Geometry: final body of the model. Coordinates: model frame, mm. A direction names the side the tool comes from. Coordinates: 2 decimals unless noted, no trailing zeros. Write each loop counter-clockwise with the first axis right and the second up, starting at its lowest first coordinate (ties: lowest second). Pieces come first, ordered by that corner, then holes. Notation, with made-up numbers: (-36.75, 33.5) -> (-28.75, 33.5) arc R33 cw to (-28.75, 71.5) -> close; hole circle Ø9 at (-35, 75.5). An arc over 180 degrees is marked (long way). One line per item, written item: value.
```python
from build123d import *

# Parameters (mm, degrees)
SKETCH1_R           = 1.5
SKETCH1_R_2         = 1.6
SKETCH1_R_3         = 2.55
SKETCH1_R_4         = 2.1
BOSS_EXTRUDE1_DEPTH = 6.25


with BuildPart() as part:
    # Sketch1 → Boss-Extrude1 (new body)
    with BuildSketch(Plane.XY):
        Polygon((180, 196.75), (-180, 196.75), (-185, 191.75), (-185, -168.25), (-180, -173.25), (-160, -173.25), (-156, -169.25), (-148, -169.25), (-144, -173.25), (-63, -173.25), (-58, -168.25), (-39, -168.25), (-34, -173.25), (144, -173.25), (148, -169.25), (156, -169.25), (160, -173.25), (180, -173.25), (185, -168.25), (185, 191.75), align=None)
        with Locations(Location((165, -153.45, 0), (0, 0, 180))):  # turned: the seam where the file's is
            Circle(SKETCH1_R, mode=Mode.SUBTRACT)
        with Locations(Location((-155, 186.55, 0), (0, 0, 180))):  # turned: the seam where the file's is
            Circle(SKETCH1_R, mode=Mode.SUBTRACT)
        with Locations(Location((-175, -133.45, 0), (0, 0, 180))):  # turned: the seam where the file's is
            Circle(SKETCH1_R, mode=Mode.SUBTRACT)
        with Locations(Location((-65, -143.25, 0), (0, 0, 180))):  # turned: the seam where the file's is
            Circle(SKETCH1_R_2, mode=Mode.SUBTRACT)
        with Locations(Location((-175, 186.55, 0), (0, 0, 180))):  # turned: the seam where the file's is
            Circle(SKETCH1_R, mode=Mode.SUBTRACT)
        with Locations(Location((-180.1, -11.45, 0), (0, 0, 180))):  # turned: the seam where the file's is
            Circle(SKETCH1_R, mode=Mode.SUBTRACT)
        with Locations(Location((-181.5, 96.05, 0), (0, 0, 180))):  # turned: the seam where the file's is
            Circle(SKETCH1_R, mode=Mode.SUBTRACT)
        with Locations(Location((-181.3, 7.85, 0), (0, 0, 180))):  # turned: the seam where the file's is
            Circle(SKETCH1_R, mode=Mode.SUBTRACT)
        with Locations(Location((-138, 1.45, 0), (0, 0, 180))):  # turned: the seam where the file's is
            Circle(SKETCH1_R, mode=Mode.SUBTRACT)
        with Locations(Location((-138.5, 96.05, 0), (0, 0, 180))):  # turned: the seam where the file's is
            Circle(SKETCH1_R, mode=Mode.SUBTRACT)
        with Locations(Location((-165, -153.45, 0), (0, 0, 180))):  # turned: the seam where the file's is
            Circle(SKETCH1_R, mode=Mode.SUBTRACT)
        with Locations(Location((-181.3, -73.45, 0), (0, 0, 180))):  # turned: the seam where the file's is
            Circle(SKETCH1_R, mode=Mode.SUBTRACT)
        with Locations(Location((175, 186.55, 0), (0, 0, 180))):  # turned: the seam where the file's is
            Circle(SKETCH1_R, mode=Mode.SUBTRACT)
        with Locations(Location((-170, 74.55, 0), (0, 0, 180))):  # turned: the seam where the file's is
            Circle(SKETCH1_R, mode=Mode.SUBTRACT)
        with Locations(Location((-138, -73.45, 0), (0, 0, 180))):  # turned: the seam where the file's is
            Circle(SKETCH1_R, mode=Mode.SUBTRACT)
        with Locations(Location((155, -133.45, 0), (0, 0, 180))):  # turned: the seam where the file's is
            Circle(SKETCH1_R, mode=Mode.SUBTRACT)
        with Locations(Location((175, -133.45, 0), (0, 0, 180))):  # turned: the seam where the file's is
            Circle(SKETCH1_R, mode=Mode.SUBTRACT)
        with Locations(Location((-180.1, -105.45, 0), (0, 0, 180))):  # turned: the seam where the file's is
            Circle(SKETCH1_R, mode=Mode.SUBTRACT)
        with Locations(Location((155, 186.55, 0), (0, 0, 180))):  # turned: the seam where the file's is
            Circle(SKETCH1_R, mode=Mode.SUBTRACT)
        with Locations(Location((-170, 117.55, 0), (0, 0, 180))):  # turned: the seam where the file's is
            Circle(SKETCH1_R, mode=Mode.SUBTRACT)
        with Locations(Location((-159, -166.25, 0), (0, 0, 180))):  # turned: the seam where the file's is
            Circle(SKETCH1_R_2, mode=Mode.SUBTRACT)
        with Locations(Location((133.6, -168.35, 0), (0, 0, 180))):  # turned: the seam where the file's is
            Circle(SKETCH1_R_3, mode=Mode.SUBTRACT)
        with Locations(Location((-145, -166.25, 0), (0, 0, 180))):  # turned: the seam where the file's is
            Circle(SKETCH1_R_2, mode=Mode.SUBTRACT)
        with Locations(Location((96.6, -145.15, 0), (0, 0, 180))):  # turned: the seam where the file's is
            Circle(SKETCH1_R_3, mode=Mode.SUBTRACT)
        with Locations(Location((73.4, -168.35, 0), (0, 0, 180))):  # turned: the seam where the file's is
            Circle(SKETCH1_R_3, mode=Mode.SUBTRACT)
        with Locations(Location((-73.4, -168.35, 0), (0, 0, 180))):  # turned: the seam where the file's is
            Circle(SKETCH1_R_3, mode=Mode.SUBTRACT)
        with Locations(Location((96.6, -168.35, 0), (0, 0, 180))):  # turned: the seam where the file's is
            Circle(SKETCH1_R_3, mode=Mode.SUBTRACT)
        with Locations(Location((-73.4, -145.15, 0), (0, 0, 180))):  # turned: the seam where the file's is
            Circle(SKETCH1_R_3, mode=Mode.SUBTRACT)
        with Locations(Location((-110.4, -168.35, 0), (0, 0, 180))):  # turned: the seam where the file's is
            Circle(SKETCH1_R_3, mode=Mode.SUBTRACT)
        with Locations(Location((-133.6, -168.35, 0), (0, 0, 180))):  # turned: the seam where the file's is
            Circle(SKETCH1_R_3, mode=Mode.SUBTRACT)
        with Locations(Location((-110.4, -145.15, 0), (0, 0, 180))):  # turned: the seam where the file's is
            Circle(SKETCH1_R_3, mode=Mode.SUBTRACT)
        with Locations(Location((73.4, -145.15, 0), (0, 0, 180))):  # turned: the seam where the file's is
            Circle(SKETCH1_R_3, mode=Mode.SUBTRACT)
        with Locations(Location((146, -166.25, 0), (0, 0, 180))):  # turned: the seam where the file's is
            Circle(SKETCH1_R_2, mode=Mode.SUBTRACT)
        with Locations(Location((-133.6, -145.15, 0), (0, 0, 180))):  # turned: the seam where the file's is
            Circle(SKETCH1_R_3, mode=Mode.SUBTRACT)
        with Locations(Location((110.4, -145.15, 0), (0, 0, 180))):  # turned: the seam where the file's is
            Circle(SKETCH1_R_3, mode=Mode.SUBTRACT)
        with Locations(Location((-96.6, -145.15, 0), (0, 0, 180))):  # turned: the seam where the file's is
            Circle(SKETCH1_R_3, mode=Mode.SUBTRACT)
        with Locations(Location((110.4, -168.35, 0), (0, 0, 180))):  # turned: the seam where the file's is
            Circle(SKETCH1_R_3, mode=Mode.SUBTRACT)
        with Locations(Location((133.6, -145.15, 0), (0, 0, 180))):  # turned: the seam where the file's is
            Circle(SKETCH1_R_3, mode=Mode.SUBTRACT)
        with Locations(Location((-96.6, -168.35, 0), (0, 0, 180))):  # turned: the seam where the file's is
            Circle(SKETCH1_R_3, mode=Mode.SUBTRACT)
        with Locations(Location((158, -166.25, 0), (0, 0, 180))):  # turned: the seam where the file's is
            Circle(SKETCH1_R_2, mode=Mode.SUBTRACT)
        with Locations(Location((-65, -160.25, 0), (0, 0, 180))):  # turned: the seam where the file's is
            Circle(SKETCH1_R_2, mode=Mode.SUBTRACT)
        with Locations(Location((-65, -169.25, 0), (0, 0, 180))):  # turned: the seam where the file's is
            Circle(SKETCH1_R_2, mode=Mode.SUBTRACT)
        with Locations(Location((45, -160.25, 0), (0, 0, 180))):  # turned: the seam where the file's is
            Circle(SKETCH1_R_2, mode=Mode.SUBTRACT)
        with Locations(Location((148.4, 31.75, 0), (0, 0, 180))):  # turned: the seam where the file's is
            Circle(SKETCH1_R_4, mode=Mode.SUBTRACT)
        with Locations(Location((45, -169.25, 0), (0, 0, 180))):  # turned: the seam where the file's is
            Circle(SKETCH1_R_2, mode=Mode.SUBTRACT)
        with Locations(Location((148.4, -85.25, 0), (0, 0, 180))):  # turned: the seam where the file's is
            Circle(SKETCH1_R_4, mode=Mode.SUBTRACT)
        with Locations(Location((-32, -160.25, 0), (0, 0, 180))):  # turned: the seam where the file's is
            Circle(SKETCH1_R_2, mode=Mode.SUBTRACT)
        with Locations(Location((-32, -169.25, 0), (0, 0, 180))):  # turned: the seam where the file's is
            Circle(SKETCH1_R_2, mode=Mode.SUBTRACT)
        with Locations(Location((-142.1, -11.45, 0), (0, 0, 180))):  # turned: the seam where the file's is
            Circle(SKETCH1_R, mode=Mode.SUBTRACT)
        with Locations(Location((-155, -133.45, 0), (0, 0, 180))):  # turned: the seam where the file's is
            Circle(SKETCH1_R, mode=Mode.SUBTRACT)
        with Locations(Location((-142.1, -105.45, 0), (0, 0, 180))):  # turned: the seam where the file's is
            Circle(SKETCH1_R, mode=Mode.SUBTRACT)
        Polygon((-92, -141.75), (-97, -136.75), (-102, -136.75), (-112, -126.75), (-130, -126.75), (-135, -121.75), (-135, 151.75), (-130, 156.75), (130, 156.75), (135, 151.75), (135, -121.75), (130, -126.75), (112, -126.75), (102, -136.75), (97, -136.75), (92, -141.75), (78, -141.75), (73, -136.75), (25, -136.75), (5, -156.75), (-5, -156.75), (-25, -136.75), (-73, -136.75), (-78, -141.75), align=None, mode=Mode.SUBTRACT)
    extrude(amount=-BOSS_EXTRUDE1_DEPTH)


solid = part.part
```
(1) Section C-C (z = -4.5). State how many separate pieces and enclosed holes the cut face has, then the cut area to 3 significant figures.
Responses:
separate pieces: 1
enclosed holes: 52
area: 56,600 mm2
(2) Section B-B (y = 22). Return the cut outline in (x, z).
Responses:
outline: (-185, -6.25) -> (-135, -6.25) -> (-135, 0) -> (-185, 0) -> close; (135, -6.25) -> (185, -6.25) -> (185, 0) -> (135, 0) -> close
(3) Line query: line 1 (Y direction, x = -175, z = -2.5); line 2 (X direction, y = -85.25, z = -2); line 3 (X direction, y = -57, z = -5.5). Output: solid intervals per line, ascending. Write a range as [from, to].
Responses:
line 1: y = [-173.25, -134.95], [-131.95, 185.05], [188.05, 196.75]
line 2: x = [-185, -135], [135, 146.3], [150.5, 185]
line 3: x = [-185, -135], [135, 185]
(4) Reachability of faces 1 (the flat face through (-3, 179, 0)), 2 (the flat face through (15.14, -146.61, -3.08)) from +Z, -Z, +X, -X, +Y, -Y: full face, straight path, thin tool, end or side. Return the list, or none.
Responses:
face 1: +Z, +X, -X, +Y, -Y
face 2: +Z, -Z
(5) Section A-A (x = 14.5). Return the cut outline in (y, z).
Responses:
outline: (-173.25, -6.25) -> (-147.25, -6.25) -> (-147.25, 0) -> (-173.25, 0) -> close; (156.75, -6.25) -> (196.75, -6.25) -> (196.75, 0) -> (156.75, 0) -> close
(6) Pull-direction query (Y, two-part tool) for faces 3 (the flat face through (-14.86, -146.89, -3.08)), 4 (the flat face through (-3, 179, -6.25)); classes: released by +Y, released by -Y, zero draft, split by the parting line, or undercut.
Responses:
face 3: undercut
face 4: zero draft
(7) First-contact query: pin 1 (2.5 mm diameter, centred on x = -180.1, y = -11.45, fed in from -Z); pin 2 (3 mm diameter, centred on x = 154, z = -2, fed in from -Y). Flat tips, straight axial feed; report the tip coordinate or a pass-through.
Responses:
pin 1: passes through
pin 2: stops at y = -169.25
